Study the drawing (mm; zero at the part's minimum x, y, z) and answer. A direction names the side the tool comes from. Round coordinates to 2 decimals unless told otherwise and drop trailing zeros. Loops run counter-clockwise (first coordinate to the right, second up) from the corner with the lowest first, then second, coordinate; pieces in that order, holes last. Notation, with made-up numbers: M 27.5,74 L 82.5,74 A17 ccw 82.5,107 Z; hole C -16,-8.5 d7. An arc over 180 degrees is marked long. Put each result on its own line as item: value. Start each with the question number.
(1) Section A-A, the plane z = 23.5 is taken. Determine the outline of the cut face in (x, y), then the cut area to 3 significant figures.
(2) Section B-B, the plane x = 89.5 is taken. Determine the outline of the cut face in (y, z), then the cut area to 3 significant figures.
(3) Which of the six approach directions +Z, -Z, +X, -X, +Y, -Y give full straight-line access (tool end or side, diameter ignored) to the marked faces 1 and 2?
(4) Section C-C, the plane y = 16 is taken. Determine the outline of the cut face in (x, z), then the cut area to 3 significant figures.
(5) Determine the mould class of the marked faces 3, 4 and 5 for opening direction Z: released by +Z, released by -Z, zero draft, split by the parting line, or undercut.
(6) Straight lines are drawn through the part: line 1 (Y direction, x = 69.5, z = 74.5); line 2 (Z direction, x = 43, y = 21.25); line 3 (Z direction, x = 84.5, y = 1.75). For each, find the intervals that lie inside material, in ascending order.
(7) Flat-ended cylindrical pins translate along their axes: P1, Ø5, axis at x = 36, z = 23, coming from the -Y side; P2, Ø6, axis at x = 79, z = 67, coming from the +Y side; P3, Ø1.5, axis at x = 99.5, z = 51, coming from the +Y side. Find the tip coordinate at first contact, or state that the pin passes through.
(8) Section D-D, the plane y = 23 is taken. Determine the outline of the cut face in (x, z), then the cut area to 3 significant figures.
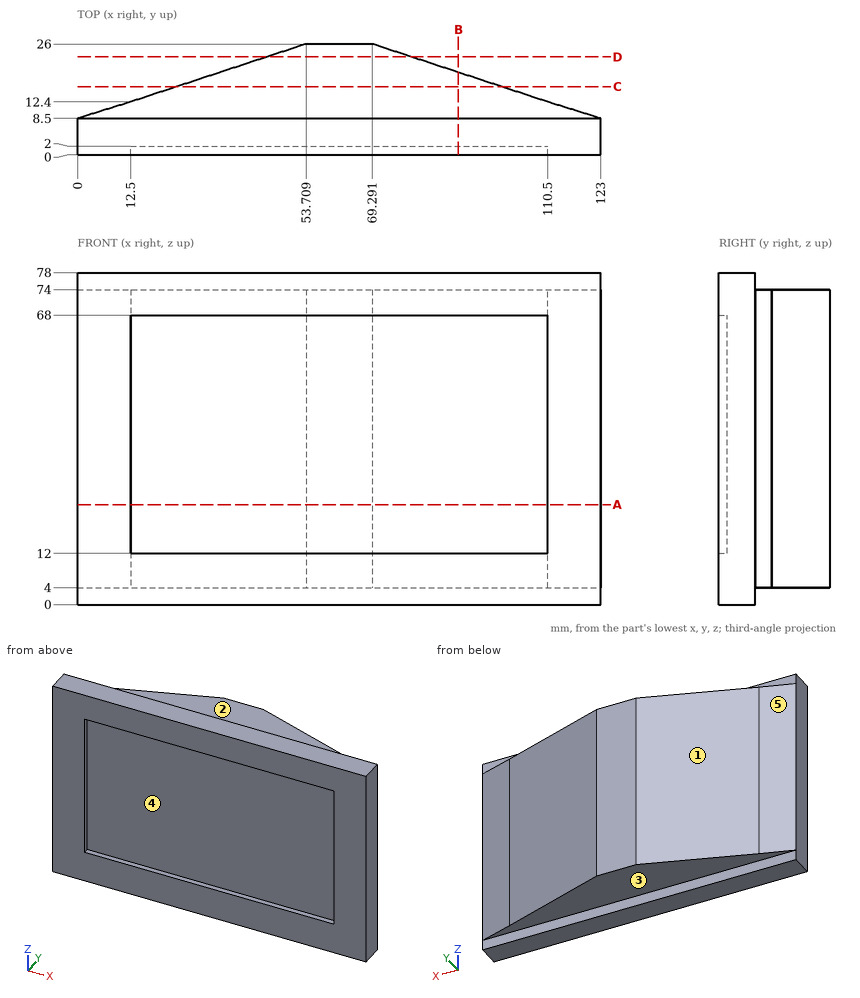
Recorded:
1. outline: M 0,0 L 12.5,0 L 12.5,2 L 110.5,2 L 110.5,0 L 123,0 L 123,8.5 L 110.5,12.4 L 69.29,26 L 53.71,26 L 12.5,12.4 L 0,8.5 Z
1. area: 2,050 mm²
2. outline: M 0,0 L 8.5,0 L 8.5,4 L 19.33,4 L 19.33,74 L 8.5,74 L 8.5,78 L 0,78 L 0,68 L 2,68 L 2,12 L 0,12 Z
2. area: 1,310 mm²
3. face 1: +Z, -Z, -X, +Y
3. face 2: +Z, +X, -X, +Y
4. outline: M 23.41,4 L 99.59,4 L 99.59,74 L 23.41,74 Z
4. area: 5,330 mm²
5. face 3: released by -Z
5. face 4: undercut
5. face 5: zero draft
6. line 1: y = 0 to 8.5
6. line 2: z = 4 to 74
6. line 3: z = 0 to 12, 68 to 78
7. P1: stops at y = 2
7. P2: stops at y = 23.79
7. P3: stops at y = 16.28
8. outline: M 44.62,4 L 78.38,4 L 78.38,74 L 44.62,74 Z
8. area: 2,360 mm²
